from build123d import *

# Parameters (mm, degrees)
F0_R     = 38.1
F1_DEPTH = 101.6
F2_R     = 34.29
F3_DEPTH = 95.25


# Not quite as in the source:
# - a fillet or chamfer that OpenCascade refuses, or shapes differently, is made with other operations: its cross-section is extruded or revolved along the edge and cut away or added


with BuildPart() as f1:
    # F0 (on Top) → F1 (new body)
    with BuildSketch(Plane.XY):
        Circle(F0_R)
    extrude(amount=F1_DEPTH)

    # F2 (on Top) → F3 (cut)
    with BuildSketch(Plane.XY):
        Circle(F2_R)
    extrude(amount=F3_DEPTH, mode=Mode.SUBTRACT)

    # F4: fillet of radius 5.08 on 2 edges, made by hand

    # F4_s1 → F4_t2 (revolve, cut)
    with BuildSketch(Plane.XZ):
        with BuildLine():
            ThreePointArc((38.1, 4.9186888497), (37.0360926284, 1.8078368763), (34.29, 0))
            Line((34.29, 0), (38.1, 0))
            Line((38.1, 0), (38.1, 4.9186888497))
        make_face()
    revolve(axis=Axis((0, 0, 0), (0, 0, 1)), mode=Mode.SUBTRACT)

    # F4_s3 → F4_t4 (revolve, cut)
    with BuildSketch(Plane.XZ):
        with BuildLine():
            ThreePointArc((38.1, 96.52), (36.6121024484, 100.1121024484), (33.02, 101.6))
            Line((33.02, 101.6), (38.1, 101.6))
            Line((38.1, 101.6), (38.1, 96.52))
        make_face()
    revolve(axis=Axis((0, 0, 101.6), (0, 0, 1)), mode=Mode.SUBTRACT)


solid = f1.part
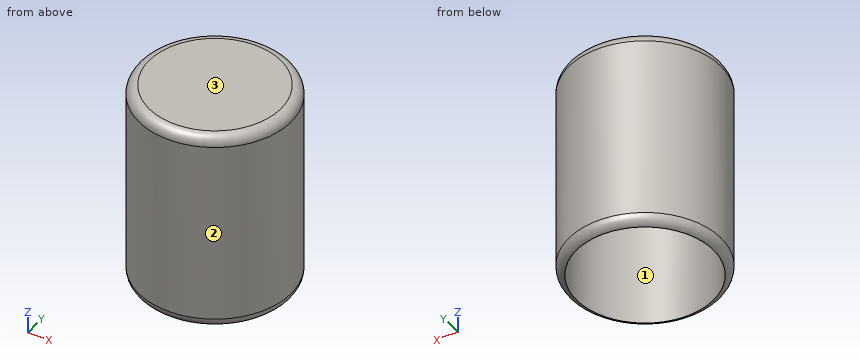
Here's how the part is built. I have some questions about the finished solid (model axes, mm). Face numbers are marked on the shaded views. Give positions to 0.01 mm unless a question says otherwise; leave off trailing zeros. Loops run counter-clockwise (first coordinate to the right, second up) from the corner with the lowest first, then second, coordinate; pieces in that order, holes last. Notation, with made-up numbers: (48, 31) -> (55, 31) arc R22 cw to (55, 44) -> close; hole circle Ø4 at (-1, -26). An arc over 180 degrees is marked (long way). Answer as a JSON object with one key per item and string values. Group by question number.
Item 1: Imagine slicing it at A-A on y = 0. Write out the boundary of the cut face in (x, z), then the cut area to 3 significant figures.
Item 2: Thinking about a two-plate mould opening in Y: for the marked faces 1, 2 and 3, which applies, pulls with the +Y half, pulls with the -Y half, needs draft (parallel to the pull), parting line crosses it, or undercut?
Item 3: I need wall thicknesses on L1, parallel to Y at x = 0, z = 80; L2, parallel to Z at x = -25.5, y = -6; L3, parallel to X at y = -1, z = 83. Which ranges of each line are inside material? Lowest first, please.
Item 4: Will these pins go through, and if not, where does the flat tip stop? pin 1 (12 mm diameter, centred on y = 27.5, z = 34.5, fed in from -X); pin 2 (3 mm diameter, centred on x = 28.5, z = 67.5, fed in from +Y); pin 3 (1 mm diameter, centred on y = 21.5, z = 80.5, fed in from -X).
Item 5: Imagine slicing it at C-C on z = 19. Write out the boundary of the cut face in (x, y), then the cut area to 3 significant figures.
Answer list:
{
 "1": {"outline": "(-38.1, 4.92) arc R5.08 ccw to (-34.29, 0) -> (-34.29, 95.25) -> (34.29, 95.25) -> (34.29, 0) arc R5.08 ccw to (38.1, 4.92) -> (38.1, 96.52) arc R5.08 ccw to (33.02, 101.6) -> (-33.02, 101.6) arc R5.08 ccw to (-38.1, 96.52) -> close", "area": "1,190 mm2"},
 "2": {"face 1": "undercut", "face 2": "parting line crosses it", "face 3": "needs draft"},
 "3": {"L1": "y = -38.1 to -34.29, 34.29 to 38.1", "L2": "z = 95.25 to 101.6", "L3": "x = -38.09 to -34.28, 34.28 to 38.09"},
 "4": {"pin 1": "stops at x = -31.45", "pin 2": "stops at y = 26.88", "pin 3": "stops at x = -31.79"},
 "5": {"outline": "circle Ø76.2 at (0, 0); hole circle Ø68.58 at (0, 0)", "area": "866 mm2"}
}
